Can you work these out from the drawing? Everything is in mm from the part's minimum corner. Coordinates: 2 decimals unless noted, no trailing zeros. Loops run counter-clockwise (first coordinate to the right, second up) from the corner with the lowest first, then second, coordinate; pieces in that order, holes last. Notation, with made-up numbers: (-37.75, -37.75) -> (6.25, -37.75) arc R7 ccw to (6.25, -32.75) -> close; hole circle Ø7 at (-15.75, 60.25). An arc over 180 degrees is marked (long way). Use one line per item in the form item = value. Start each with the question number.
(1) Imagine slicing it at B-B (y = 110). List the corners of the cut face in (x, z) for me.
(2) I'm going to push flat-ended pins straight in: pin 1 (4 mm diameter, centred on x = 106.5, z = 2.5, fed in from -Y) (1 decimal); pin 2 (2.5 mm diameter, centred on x = 107.5, z = 6, fed in from -Y); pin 3 (2.5 mm diameter, centred on x = 105.5, z = 4.5, fed in from -Y); pin 4 (1.5 mm diameter, centred on x = 31.5, y = 69, fed in from -Z). Where does each tip first touch, or does it pass through?
(3) Imagine slicing it at A-A (z = 2.5). List the corners of the cut face in (x, y) for me, plus the area to 3 significant figures.
(4) Imagine slicing it at C-C (x = 88). List the corners of the cut face in (y, z) for me (1 decimal).
(5) I need wall thicknesses on line 1 (X direction, y = 160, z = 5); line 2 (X direction, y = 142.5, z = 0.5); line 3 (Y direction, x = 17.5, z = 0.75). Which ranges of each line are inside material? Lowest first, please. Write a range as [from, to].
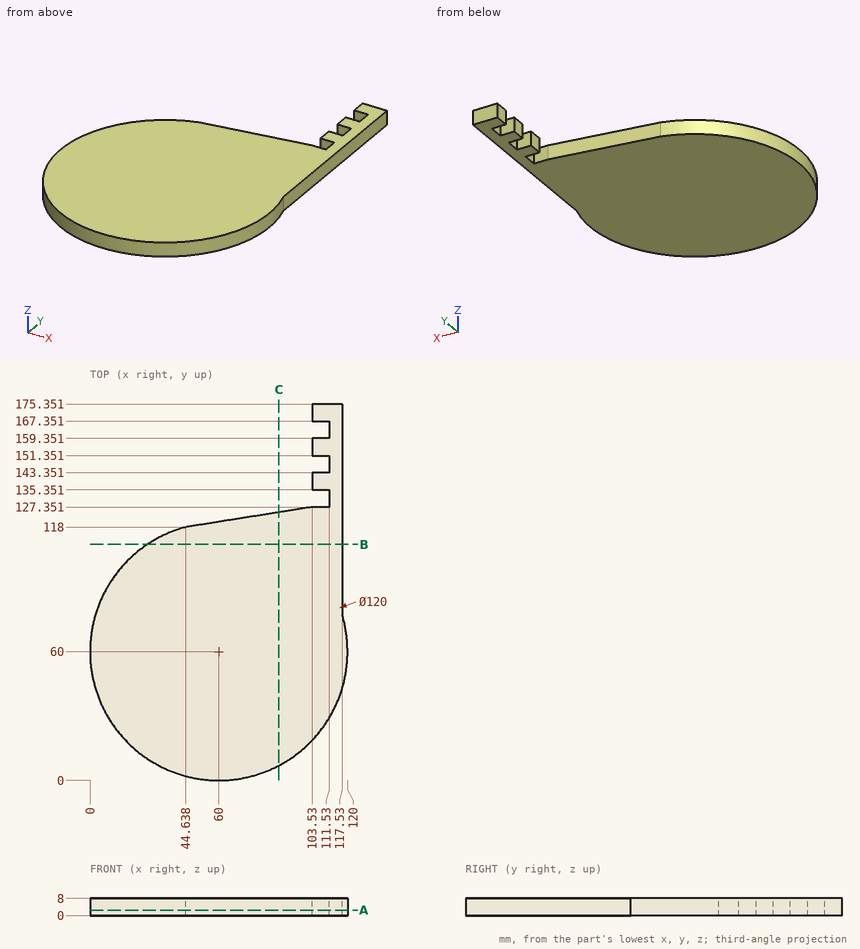
Worked out:
q1.outline = (26.83, 0) -> (117.53, 0) -> (117.53, 8) -> (26.83, 8) -> close
q2.pin_1 = 19.8
q2.pin_2 = 21.78
q2.pin_3 = 19.48
q2.pin_4 = 0
q3.outline = (44.64, 118) arc R60 ccw (long way) to (117.53, 77.04) -> (117.53, 175.35) -> (103.53, 175.35) -> (103.53, 167.35) -> (111.53, 167.35) -> (111.53, 159.35) -> (103.53, 159.35) -> (103.53, 151.35) -> (111.53, 151.35) -> (111.53, 143.35) -> (103.53, 143.35) -> (103.53, 135.35) -> (111.53, 135.35) -> (111.53, 127.35) -> (103.53, 127.35) -> close
q3.area = 12,700 mm2
q4.outline = (6.9, 0) -> (124.9, 0) -> (124.9, 8) -> (6.9, 8) -> close
q5.line_1 = [111.53, 117.53]
q5.line_2 = [103.53, 117.53]
q5.line_3 = [17.65, 102.35]
